Input: dimensioned drawing with shaded views. Units: mm. Origin: part minimum x, y, z. A direction names the side the tool comes from. Round coordinates to 2 decimals unless told otherwise and drop trailing zeros. Loops run counter-clockwise (first coordinate to the right, second up) from the corner with the lowest first, then second, coordinate; pieces in that order, holes last. Notation, with made-up numbers: M 5,-11.75 L 13,-11.75 A23 ccw 13,14.25 Z; hole C 9,-18 d8. An arc over 180 degrees is marked long. One line per item, written item: value.
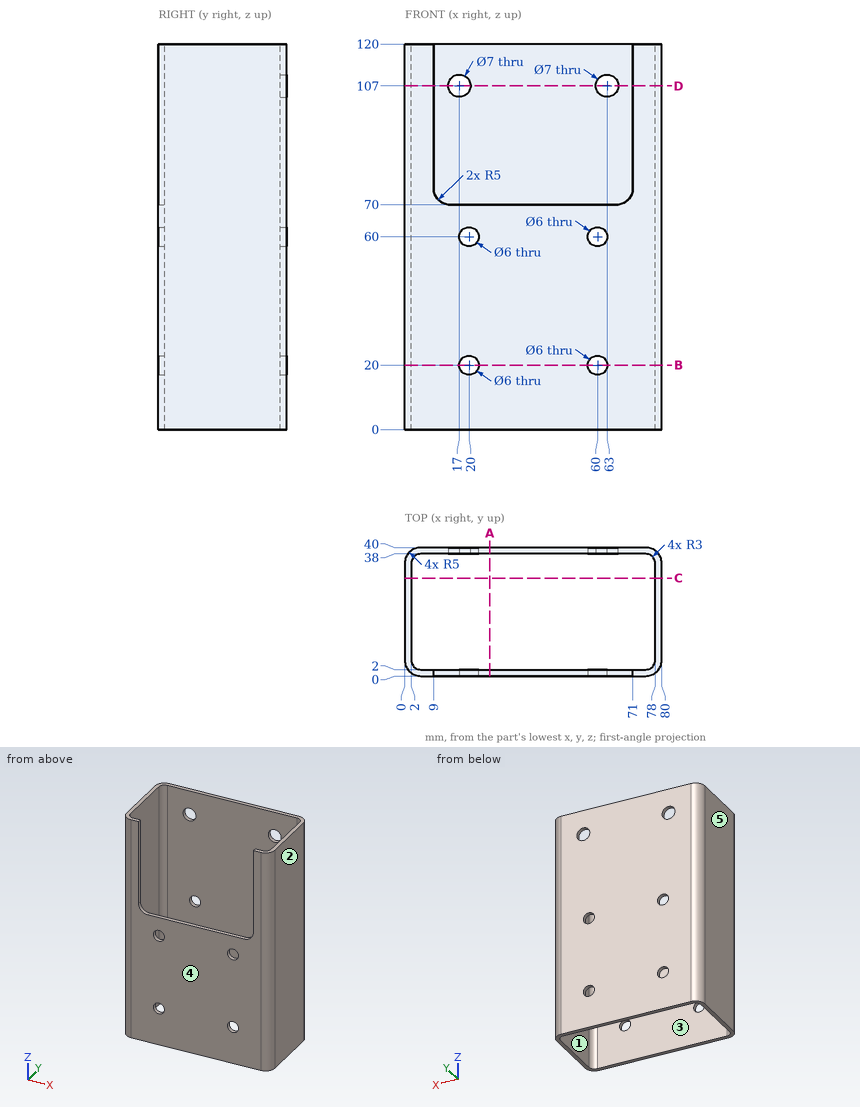
1. Section query B-B (z = 20). Count the separate pieces of the cut face and the enclosed holes in it, and give its area (3 significant figures).
Report:
separate pieces: 4
enclosed holes: 0
area: 402 mm2
2. Pull-direction query (X, two-part tool) for the marked faces 3, 4 and 5; classes: released by +X, released by -X, zero draft, split by the parting line, or undercut.
Report:
face 3: undercut
face 4: zero draft
face 5: released by -X
3. Section query C-C (y = 30.5). Return the cut outline in (x, z), and give its area (3 significant figures).
Report:
outline: M 0,0 L 2,0 L 2,120 L 0,120 Z; M 78,0 L 80,0 L 80,120 L 78,120 Z
area: 480 mm2
4. Reachability of the marked faces 1 and 2 from +Z, -Z, +X, -X, +Y, -Y: full face, straight path, thin tool, end or side. Return the list, or none.
Report:
face 1: +Z, -Z
face 2: +Z, -Z, +X, +Y, -Y
5. Section query A-A (x = 26.5). Return the cut outline in (y, z).
Report:
outline: M 0,0 L 2,0 L 2,70 L 0,70 Z; M 38,0 L 40,0 L 40,120 L 38,120 Z
6. Ray query, line 1 (Z direction, x = 60, y = 1); line 2 (X direction, y = 19, z = 8.5); line 3 (Y direction, x = 20, z = 51). Return the intervals inside material, ascending. Write a range as [from, to].
Report:
line 1: z = [0, 17], [23, 57], [63, 70]
line 2: x = [0, 2], [78, 80]
line 3: y = [0, 2], [38, 40]
7. Section query D-D (z = 107). Return the cut outline in (x, y).
Report:
outline: M 0,5 A5 ccw 5,0 L 9,0 L 9,2 L 5,2 A3 cw 2,5 L 2,35 A3 cw 5,38 L 13.5,38 L 13.5,40 L 5,40 A5 ccw 0,35 Z; M 20.5,38 L 59.5,38 L 59.5,40 L 20.5,40 Z; M 66.5,38 L 75,38 A3 cw 78,35 L 78,5 A3 cw 75,2 L 71,2 L 71,0 L 75,0 A5 ccw 80,5 L 80,35 A5 ccw 75,40 L 66.5,40 Z
8. Pin query (flat end, axial travel): pin 1 (1.6 mm diameter, centred on y = 1, z = 95.5, fed in from -X); pin 2 (3.5 mm diameter, centred on x = 20, z = 20, fed in from -Y); pin 3 (0.6 mm diameter, centred on y = 1.5, z = 108, fed in from +X); pin 4 (4 mm diameter, centred on x = 10.5, z = 30.5, fed in from -Y). Return the tip coordinate at first contact, or that it passes through.
Report:
pin 1: stops at x = 1.16
pin 2: passes through
pin 3: stops at x = 78.84
pin 4: stops at y = 0
